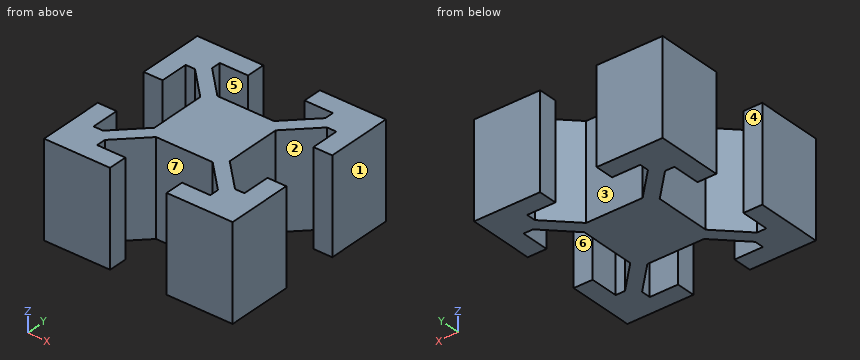
from build123d import *

# Parameters (mm, degrees)
PAD_DEPTH    = 10
SKETCH001_R  = 2
POCKET_DEPTH = 4.001


with BuildPart() as change_me_for_height:
    # Sketch → Pad (new body)
    with BuildSketch(Plane.XY):
        Polygon((-10, 3), (-10, 10), (-3, 10), (-3, 8), (-6, 8), (-6, 7), (-3, 4), (3, 4), (6, 7), (6, 8), (3, 8), (3, 10), (10, 10), (10, 3), (8, 3), (8, 6), (7, 6), (4, 3), (4, 0), (-4, 0), (-4, 3), (-7, 6), (-8, 6), (-8, 3), align=None)
    pad = extrude(amount=PAD_DEPTH)


with BuildPart() as mirrored:
    # Mirrored base: copy of Change_me_for_height
    add(change_me_for_height.part)

    # Mirrored: Pad across Sketch H_Axis
    add(pad.mirror(Plane.ZX))


with BuildPart() as pocket:
    # Fusion base: copy of Change_me_for_height
    add(change_me_for_height.part)

    # Fusion: union Mirrored
    add(mirrored.part)

    # Sketch001 → Pocket (cut, through all)
    with BuildSketch(Plane.XZ.offset(-6)):
        Circle(SKETCH001_R)
    extrude(amount=-POCKET_DEPTH, mode=Mode.SUBTRACT)


solid = pocket.part
Verification items for the finished model (mm, model axes). Face numbers are marked on the shaded views. A direction names the side the tool comes from. Give positions to 0.01 mm unless a question says otherwise; leave off trailing zeros. Order: outer loops, then holes, each group sorted by start corner. A loop starts at its lowest first (then second) coordinate and runs counter-clockwise, first axis right, second up. Notation, with made-up numbers: M -37,50.5 L -19,50.5 A21 ccw -19,61.5 Z; hole C 78,46.25 d8. An arc over 180 degrees is marked long. Use one line per item in the form item = value. Start each with the question number.
Q1. Section check C-C (y = 8.5). Enter the section's corners in (x, z).
Q2. Section check B-B (x = -6.5). Enter the section's corners in (y, z), then the cut area to 3 significant figures.
Q3. Mould release check, pull along Y, two halves, no side actions. Record for the marked faces 1, 2 and 3: +Y half, -Y half, draft (parallel to the pull), parting line (faces both ways), or undercut.
Q4. Section check A-A (y = 3.5). Enter the section's corners in (x, z).
Q5. Access from +Z, -Z, +X, -X, +Y, -Y to the whole of each face (thin tool, end or side, straight path). Record for the marked faces 4, 5, 6 and 7.
Q6. Section check D-D (x = 5.75). Enter the section's corners in (y, z).
Q7. Scan lines: line 1 along Y through (x, z) = (5, 2.5); line 2 along X through (y, z) = (8.5, 3.5); line 3 along X through (y, z) = (-4.5, 3.5). Record each from-to range of solid material in increasing order. Write a range as [from, to].
Q8. Go/stop test with flat-tipped pins: pin 1 Ø8 at (x, y) = (-2.5, -7) entering from +Z; pin 2 Ø1 at (x, z) = (-1, 3) entering from -Y; pin 3 Ø1.8 at (y, z) = (-0.5, 5.5) entering from -X. Record where each tip stops, or that it passes through.
Evaluation:
q1.outline = M -10,0 L -3,0 L -3,10 L -10,10 Z; M 3,0 L 10,0 L 10,10 L 3,10 Z
q2.outline = M -10,0 L -5.5,0 L -5.5,10 L -10,10 Z; M 5.5,0 L 10,0 L 10,10 L 5.5,10 Z
q2.area = 90.0 mm2
q3.face_1 = draft
q3.face_2 = undercut
q3.face_3 = +Y half
q4.outline = M -10,0 L -8,0 L -8,10 L -10,10 Z; M -4.5,0 L 4.5,0 L 4.5,10 L -4.5,10 Z; M 8,0 L 10,0 L 10,10 L 8,10 Z
q5.face_4 = +Z, -Z, -X
q5.face_5 = +Z, -Z
q5.face_6 = +Z, -Z, +X
q5.face_7 = +Z, -Z, -Y
q6.outline = M -10,0 L -8,0 L -8,10 L -10,10 Z; M -6.75,0 L -4.75,0 L -4.75,10 L -6.75,10 Z; M 4.75,0 L 6.75,0 L 6.75,10 L 4.75,10 Z; M 8,0 L 10,0 L 10,10 L 8,10 Z
q7.line_1 = [-10, -8], [-6, -4], [4, 6], [8, 10]
q7.line_2 = [-10, -3], [3, 10]
q7.line_3 = [-10, -8], [-5.5, -3.5], [3.5, 5.5], [8, 10]
q8.pin_1 = 10
q8.pin_2 = -4
q8.pin_3 = -4
